from build123d import *

# Parameters (mm, degrees)
BOSS_EXTRUDE7_DEPTH = 139
CUT_EXTRUDE1_DEPTH  = 19
CUT_EXTRUDE2_DEPTH  = 19
FILLET5_R           = 2
FILLET6_R           = 2
SKETCH11_R          = 3.75
CUT_EXTRUDE3_DEPTH  = 121
CUT_EXTRUDE4_DEPTH  = 41
CUT_EXTRUDE5_DEPTH  = 10
FILLET7_R           = 1


with BuildPart() as part:
    # Sketch1 → Boss-Extrude7 (new body)
    with BuildSketch(Plane.XY):
        with BuildLine():
            Line((0, 10), (0, 40))
            ThreePointArc((0, 40), (-28.284271247, -28.284271247), (40, 0))
            Line((40, 0), (0, 0))
            Line((0, 0), (0, 4))
            Line((0, 4), (-12, 4))
            ThreePointArc((-12, 4), (-15, 7), (-12, 10))
            Line((-12, 10), (0, 10))
        make_face()
    extrude(amount=BOSS_EXTRUDE7_DEPTH)

    # Sketch8 → Cut-Extrude1 (cut)
    with BuildSketch(Plane.XY.offset(139)):
        with BuildLine():
            Line((25, 0), (40, 0))
            ThreePointArc((40, 0), (-28.284271247, -28.284271247), (0, 40))
            Line((0, 40), (0, 25))
            ThreePointArc((0, 25), (-17.67766953, -17.67766953), (25, 0))
        make_face()
    extrude(amount=-CUT_EXTRUDE1_DEPTH, mode=Mode.SUBTRACT)

    # Sketch9 → Cut-Extrude2 (cut)
    with BuildSketch(Plane(origin=(0, 0, 0), x_dir=(-1, 0, 0), z_dir=(0, 0, -1))):
        with BuildLine():
            Line((-25, 0), (-40, 0))
            ThreePointArc((-40, 0), (28.284271247, -28.284271247), (0, 40))
            Line((0, 40), (0, 25))
            ThreePointArc((0, 25), (17.67766953, -17.67766953), (-25, 0))
        make_face()
    extrude(amount=-CUT_EXTRUDE2_DEPTH, mode=Mode.SUBTRACT)

    # Fillet5
    fillet5_edges = [part.edges().sort_by_distance(p)[0] for p in [
        (-17.67766953, -17.67766953, 120),
    ]]
    fillet(fillet5_edges, radius=FILLET5_R)

    # Fillet6
    fillet6_edges = [part.edges().sort_by_distance(p)[0] for p in [
        (-17.67766953, -17.67766953, 19),
    ]]
    fillet(fillet6_edges, radius=FILLET6_R)

    # Sketch10 → Cut-Revolve6 (revolve, cut)
    with BuildSketch(Plane(origin=(0, 0, 0), x_dir=(0, 0, -1), z_dir=(1, 0, 0))):
        Polygon((-47.5, 40), (-50, 37.5), (-89, 37.5), (-91.5, 40), align=None)
    revolve(axis=Axis((0, 0, 139), (0, 0, -1)), mode=Mode.SUBTRACT)

    # Sketch11 → Cut-Extrude3 (cut, through all)
    with BuildSketch(Plane.XY.offset(120)):
        with Locations((-8.282209443, 30.909626441)):
            Circle(SKETCH11_R)
        with Locations((30.909626441, -8.282209443)):
            Circle(SKETCH11_R)
        with Locations((22.627416998, -22.627416998)):
            Circle(SKETCH11_R)
        with Locations((8.282209443, -30.909626441)):
            Circle(SKETCH11_R)
        with Locations((-8.282209443, -30.909626441)):
            Circle(SKETCH11_R)
        with Locations((-22.627416998, -22.627416998)):
            Circle(SKETCH11_R)
        with Locations((-30.909626441, -8.282209443)):
            Circle(SKETCH11_R)
        with Locations((-30.909626441, 8.282209443)):
            Circle(SKETCH11_R)
        with Locations((-22.627416998, 22.627416998)):
            Circle(SKETCH11_R)
    extrude(amount=-CUT_EXTRUDE3_DEPTH, mode=Mode.SUBTRACT)

    # Sketch12 → Cut-Extrude4 (cut, through all)
    with BuildSketch(Plane(origin=(0, 0, 0), x_dir=(1, 0, 0), z_dir=(0, 1, 0))):
        with BuildLine():
            Line((25, -17), (25, 0))
            Line((25, 0), (10, 0))
            ThreePointArc((10, 0), (10.114159057, -2.614672282), (10.45576741, -5.20944533))
            ThreePointArc((10.45576741, -5.20944533), (16.199399791, -18.26284287), (27.321452148, -27.189233611))
            ThreePointArc((27.321452148, -27.189233611), (33.506811582, -29.288880214), (40, -30))
            Line((40, -30), (40, -19))
            Line((40, -19), (27, -19))
            ThreePointArc((27, -19), (25.585786438, -18.414213562), (25, -17))
        make_face()
        with BuildLine():
            ThreePointArc((27.321452148, -27.189233611), (16.199399791, -18.26284287), (10.45576741, -5.20944533))
            Line((10.45576741, -5.20944533), (5.531728645, -6.077686218))
            ThreePointArc((5.531728645, -6.077686218), (12.23263309, -21.306650015), (25.208360839, -31.720772546))
            Line((25.208360839, -31.720772546), (27.321452148, -27.189233611))
        make_face()
    extrude(amount=-CUT_EXTRUDE4_DEPTH, mode=Mode.SUBTRACT)

    # Sketch16 → Cut-Extrude5 (cut)
    with BuildSketch(Plane.XY.offset(139)):
        with BuildLine():
            Line((20.615528128, -4), (-4, -4))
            Line((-4, -4), (-4, 0))
            Line((-4, 0), (-21, 0))
            ThreePointArc((-21, 0), (-2.009217424, -20.903661051), (20.615528128, -4))
        make_face()
    extrude(amount=-CUT_EXTRUDE5_DEPTH, mode=Mode.SUBTRACT)

    # Fillet7
    fillet7_edges = [part.edges().sort_by_distance(p)[0] for p in [
        (-2.009217424, -20.903661051, 129),
        (20.615528128, -4, 134),
        (-12.5, 0, 129),
        (-21, 0, 134),
        (-4, -2, 129),
        (-4, 0, 134),
        (8.307764064, -4, 129),
        (-4, -4, 134),
        (-2.009217424, -20.903661051, 139),
        (8.307764064, -4, 139),
        (-4, -2, 139),
        (-12.5, 0, 139),
    ]]
    fillet(fillet7_edges, radius=FILLET7_R)


solid = part.part
Work out the finished part from the listing and answer in its coordinate system (mm). A direction names the side the tool comes from. Give positions to 0.01 mm unless a question says otherwise; leave off trailing zeros. Write each loop counter-clockwise with the first axis right and the second up, starting at its lowest first coordinate (ties: lowest second). Pieces come first, ordered by that corner, then holes.
Q1. The part is cut by section B-B on z = 23. Give the vertices of the cut face in (x, y).
Answer:
outline: (-12, 4) arc R3 cw to (-12, 10) - (0, 10) - (0, 40) arc R40 ccw (long way) to (13.62, -37.61) - (13.62, 0) - (0, 0) - (0, 4) - close; hole circle Ø7.5 at (-30.91, -8.28); hole circle Ø7.5 at (-30.91, 8.28); hole circle Ø7.5 at (-22.63, -22.63); hole circle Ø7.5 at (-22.63, 22.63); hole circle Ø7.5 at (-8.28, -30.91); hole circle Ø7.5 at (-8.28, 30.91); hole circle Ø7.5 at (8.28, -30.91)
Q2. For a pull along Z with two mould halves and no side action, classify faces 5 (the face through (12, -15, 21)), 6 (the face through (-1, -10, 129)), 7 (the face through (-6, 10, 69)) as released by +Z, released by -Z, zero draft, split by the parting line, or undercut.
Answer:
face 5: undercut
face 6: released by +Z
face 7: zero draft
Q3. Straight lines are drawn through the part: L1, parallel to X at y = -21, z = 67.5; L2, parallel to Y at x = -29.5, z = 84; L3, parallel to Y at x = -33.5, z = 104. For each, find the intervals that lie inside material, in ascending order.
Answer:
L1: x = -31.07 to -26.01, -19.25 to 19.25, 26.01 to 31.07
L2: y = -23.15 to -11.76, -4.81 to 4.81, 11.76 to 23.15
L3: y = -21.86 to -10.99, -5.57 to 5.57, 10.99 to 21.86
Q4. A tool of negligible diameter and unlimited length cuts with its end or side. For faces 1 (the face through (-25.734, -27.491, 89.156)), 2 (the face through (26.25, -15.31, 29.49)), 3 (the face through (16, 0, 84)), 4 (the face through (-18, -21, 120)), from which of +Z, -Z, +X, -X, +Y, -Y can it reach the whole face along a straight path? Write none if from no direction.
Answer:
face 1: none
face 2: -Z, +Y, -Y
face 3: +Z, -Z, +X, +Y
face 4: +Z
Q5. The part is cut by section A-A on z = 62.5. State how many separate pieces and enclosed holes the cut face has, and give its area (3 significant figures).
Answer:
separate pieces: 1
enclosed holes: 9
area: 2,830 mm2
Q6. Given pin 1 (1.5 mm diameter, centred on y = -20.5, z = 25, fed in from +X); pin 2 (8.5 mm diameter, centred on x = 30.91, y = -8.28, fed in from +Z); pin 3 (0.6 mm diameter, centred on y = -2, z = 133, fed in from -X); pin 4 (7 mm diameter, centred on x = -8.28, y = 30.91, fed in from +Z), each flat-ended and moving along its own axis, determine where each tip first touches the part or whether it passes through.
Answer:
pin 1: stops at x = 16.29
pin 2: stops at z = 120
pin 3: stops at x = -24.94
pin 4: passes through
